from build123d import *

# Parameters (mm, degrees)
F0_R     = 12.7
F1_DEPTH = 6.35


with BuildPart() as f1:
    # F0 (on Front) → F1 (new body, symmetric)
    with BuildSketch(Plane.XZ):
        with BuildLine():
            Line((5.58851, -28.415137), (16.496631, -9.526996))
            ThreePointArc((16.496631, -9.526996), (0, 19.05), (-16.496631, -9.526996))
            Line((-16.496631, -9.526996), (-5.58851, -28.415137))
            ThreePointArc((-5.58851, -28.415137), (0, -31.75), (5.58851, -28.415137))
        make_face()
        Circle(F0_R, mode=Mode.SUBTRACT)
    extrude(amount=F1_DEPTH, both=True)


solid = f1.part
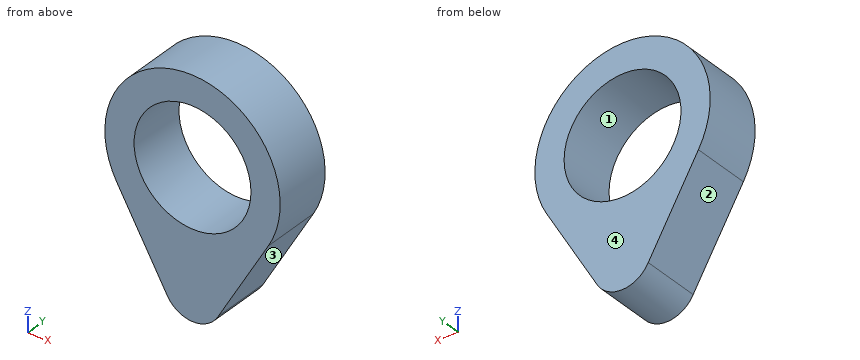
Can you work these out from the model? Positions are in its coordinate system, mm. Face numbers are marked on the shaded views. Round coordinates to 2 decimals unless told otherwise and drop trailing zeros. Write each loop counter-clockwise with the first axis right and the second up, starting at its lowest first coordinate (ties: lowest second). Pieces come first, ordered by that corner, then holes. Notation, with made-up numbers: (21.25, -19) -> (54.25, -19) arc R23 cw to (54.25, 8) -> close; hole circle Ø11 at (45, -12.75). An arc over 180 degrees is marked (long way). Use one line per item in the form item = value. Start each with the question number.
Q1. Imagine slicing it at A-A (x = 0). Please give me the cut outline in (y, z), then the cut area to 3 significant figures.
Q2. I'm going to push flat-ended pins straight in: P1, Ø2, axis at x = 0.5, z = 11, coming from the +Y side; P2, Ø2, axis at x = -2, y = 2, coming from the +Z side; P3, Ø3, axis at y = 0.5, z = -15, coming from the +X side; P4, Ø6, axis at y = 1.5, z = 1, coming from the +X side. Where does each tip first touch, or does it pass through?
Q3. Imagine slicing it at B-B (z = 0). Please give me the cut outline in (x, y).
Q4. If I drill on probe 1 along Z at (x, y) = (-4.5, 4.25); probe 2 along Z at (x, y) = (-8, 4.25); probe 3 along X at (y, z) = (1, -10), over which ranges is the centre line in solid material (lowest first)? Write a range as [from, to].
Q5. Imagine slicing it at D-D (z = -22.5). Please give me the cut outline in (x, y).
Q6. We'd pull the mould along X, two halves only. Please class the marked faces 1, 2, 3 and 4: +X half, -X half, draft (parallel to the pull), parting line (faces both ways), or undercut.
Q7. Imagine slicing it at C-C (y = -4). Please give me the cut outline in (x, z), then the cut area to 3 significant figures.
Worked out:
q1.outline = (-6.35, -31.75) -> (6.35, -31.75) -> (6.35, -12.7) -> (-6.35, -12.7) -> close; (-6.35, 12.7) -> (6.35, 12.7) -> (6.35, 19.05) -> (-6.35, 19.05) -> close
q1.area = 323 mm^2
q2.P1 = through
q2.P2 = 19.02
q2.P3 = 14.2
q2.P4 = 19.05
q3.outline = (-19.05, -6.35) -> (-12.7, -6.35) -> (-12.7, 6.35) -> (-19.05, 6.35) -> close; (12.7, -6.35) -> (19.05, -6.35) -> (19.05, 6.35) -> (12.7, 6.35) -> close
q4.probe_1 = [-29.88, -11.88], [11.88, 18.51]
q4.probe_2 = [-24.24, -9.86], [9.86, 17.29]
q4.probe_3 = [-16.22, -7.83], [7.83, 16.22]
q5.outline = (-9, -6.35) -> (9, -6.35) -> (9, 6.35) -> (-9, 6.35) -> close
q6.face_1 = undercut
q6.face_2 = -X half
q6.face_3 = +X half
q6.face_4 = draft
q7.outline = (-16.5, -9.53) -> (-5.59, -28.42) arc R6.35 ccw to (5.59, -28.42) -> (16.5, -9.53) arc R19.05 ccw (long way) to start; hole circle Ø25.4 at (0, 0)
q7.area = 854 mm^2
